Autodesk Inventor part; units mm, degrees
ref_plane "YZ Plane" through (0, 0, 0) normal (1, 0, 0) x (0, 1, 0)
ref_plane "XZ Plane" through (0, 0, 0) normal (0, 1, 0) x (-1, 0, 0)
ref_plane "XY Plane" through (0, 0, 0) normal (0, 0, 1) x (1, 0, 0)
sketch "Sketch1" plane through (0, 0, 0) normal (0, 0, 1) x (1, 0, 0)
  line L0 (0, 0) -> (103.505, 0)
  line L1 (103.505, 0) -> (103.505, -19.05)
  line L2 (103.505, -19.05) -> (0, -19.05)
  line L3 (0, -19.05) -> (0, 0)
  line L4 (19.05, 0) -> (19.05, -101.6)
  circle A0 centre (28.575, -101.6) radius 9.525
  line L5 (103.505, 0) -> (36.6455, -106.659)
  circle A1 centre (28.575, -101.6) radius 3.175
  circle A2 centre (9.525, -9.525) radius 3.175
  dimension "d0" = 103.505
  dimension "d1" = 19.05
  dimension "d2" = 101.6
  dimension "d3" = 6.35
  dimension "d4" = 6.35
extrude "Extrusion1" add sketch "Sketch1" along normal blind 3.175
sketch "Sketch2" plane through (0, 0, 3.175) normal (0, 0, 1) x (1, 0, 0)
  line L0 (91.5634, -19.05) -> (103.505, 0)
  line L1 (103.505, 0) -> (141.6118, -29.0679)
  line L2 (141.6118, -29.0679) -> (106.1951, -49.8481)
  line L3 (106.1951, -49.8481) -> (91.5634, -19.05)
  point P0 (0, 0)
extrude "Extrusion2" cut sketch "Sketch2" against normal blind 6.35
sketch "Sketch3" plane through (0, 0, 3.175) normal (0, 0, 1) x (1, 0, 0)
  line L0 (19.05, -19.05) -> (22.3566, -51.6435)
  line L1 (22.3566, -51.6435) -> (19.05, -54.458)
  line L2 (19.05, -54.458) -> (19.05, -19.05)
  line L3 (0, -19.05) -> (19.05, -19.05)
  point P0 (0, 0)
extrude "Extrusion3" cut sketch "Sketch3" against normal blind 3.175
properties part number "Elevator Latch"
Geometry: final body of the model. Coordinates: model frame, mm. A direction names the side the tool comes from. Round coordinates to 2 decimals unless told otherwise and drop trailing zeros. Write each loop counter-clockwise with the first axis right and the second up, starting at its lowest first coordinate (ties: lowest second). Pieces come first, ordered by that corner, then holes. Notation, with made-up numbers: M 18.25,-29.5 L 50.25,-29.5 A28 cw 50.25,1.5 Z; hole C -5.5,-30.75 d6. An arc over 180 degrees is marked long. Write item = value, one per line.
Item 1: Access query for faces 1 (the face through (51, -30, 3.175)), 2 (the face through (19.05, -78, 2)), 3 (the face through (20.68, -35.12, 1.61)). Directions: +Z, -Z, +X, -X, +Y, -Y. A direction counts if a zero-diameter tool reaches every point of the face in a straight line with its end or side. Return the directions, or none.
Findings:
face_1 = +Z, +X, -X, +Y, -Y
face_2 = +Z, -Z, -X, -Y
face_3 = +Z, -Z, -X
Item 2: Pull-direction query (X, two-part tool) for faces 4 (the face through (11.232, -12.202, 1.565)), 5 (the face through (10, -19.05, 2)), 6 (the face through (20.73, -53.03, 1.61)); classes: pulls with the +X half, pulls with the -X half, needs draft (parallel to the pull), parting line crosses it, or undercut.
Findings:
face_4 = undercut
face_5 = needs draft
face_6 = pulls with the -X half
Item 3: Section query A-A on z = 0.8. State how many separate pieces and enclosed holes the cut face has, then the cut area to 3 significant figures.
Findings:
separate_pieces = 1
enclosed_holes = 2
area = 5,730 mm^2
Item 4: Section query B-B on x = 61. Return loops of the section in (y, z) (3 decimals).
Findings:
outline = M -67.807,0 L 0,0 L 0,3.175 L -67.807,3.175 Z
Item 5: Material intervals for line 1 along Y through (x, z) = (17, 0.3); line 2 along Y through (x, z) = (12, 2.05); line 3 along X through (y, z) = (-31.5, 1.9), sorted ascending. Write a range as [from, to].
Findings:
line_1 = [-19.05, 0]
line_2 = [-19.05, -11.51], [-7.54, 0]
line_3 = [20.31, 83.76]
Item 6: Pin query (flat end, axial travel): P1, Ø1, axis at y = -86.5, z = 1, coming from the -X side; P2, Ø1, axis at x = 8, z = 1.5, coming from the -Y side. Return the tip coordinate at first contact, or that it passes through.
Findings:
P1 = 19.05
P2 = -19.05
